The model under review builds one solid part; all positions refer to its coordinate system, in mm. A direction names the side the tool comes from. Coordinates: 2 decimals unless noted, no trailing zeros. Write each loop counter-clockwise with the first axis right and the second up, starting at its lowest first coordinate (ties: lowest second). Pieces come first, ordered by that corner, then holes. Notation, with made-up numbers: (33.25, 50.5) - (82.25, 50.5) arc R26 ccw to (82.25, 85.5) - close; hole circle Ø10 at (-35, 71.5). An arc over 180 degrees is marked (long way). Return JSON: item names as keys, results as strings. Group by question number.
(1) For pin 1 Ø1 at (x, z) = (5.5, 4) entering from -Y; pin 2 Ø1.5 at (x, z) = (-4, 5) entering from -Y; pin 3 Ø1.8 at (y, z) = (0, 1.5) entering from +X, all flat-tipped, find the tip position at first contact; note any pin that passes through.
(2) We need section D-D on x = 10.75. State the section outline as (y, z) points, then the cut area to 3 significant figures.
(3) Draft analysis for pull direction Y (two halves, no side actions). For faces 1 (the face through (6, -13, 0)), 2 (the face through (3.715, -19.396, 2.958)), 3 (the face through (15.62, -31.28, 3.04)), 4 (the face through (5.14, -47.3, 2.96)), state which applies: released by +Y, released by -Y, zero draft, split by the parting line, or undercut.
(4) We need section C-C on z = 1.05. State the section outline as (x, y) points.
(5) To check wall thickness, follow L1, parallel to Y at x = -1.25, z = 0.3; L2, parallel to X at y = -0.5, z = 0.7; L3, parallel to X at y = -13.5, z = 4. State the ranges of each line that lie inside material, in increasing order. Write a range as from..to.
(6) We need section A-A on x = 4.5. State the section outline as (y, z) points.
(7) Tool access review of faces 5 (the face through (3.93, -41.9, 2.96)), 6 (the face through (6, -13, 6)), 7 (the face through (0, 1.778, 3)): name each direction out of +Z, -Z, +X, -X, +Y, -Y from which nothing blocks a thin tool from reaching the whole face with its end or side.
(8) We need section B-B on y = 0. State the section outline as (x, z) points, then the cut area to 3 significant figures.
Autodesk Fusion 360 part; units mm, degrees
sketch "Sketch1" plane through (0, 0, 0) normal (0, 0, 1) x (1, 0, 0)
  circle A0 centre (0, 0) radius 10
  line L0 (-1.778, 1.778) -> (1.778, 1.778)
  line L1 (1.778, 1.778) -> (1.778, -1.778)
  line L2 (1.778, -1.778) -> (-1.778, -1.778)
  line L3 (-1.778, -1.778) -> (-1.778, 1.778)
  line L4 (-1.778, 1.778) -> (1.778, -1.778) construction
  line L5 (1.778, 1.778) -> (-1.778, -1.778) construction
  line L6 (0, 10) -> (0, -50.96)
  line L7 (0, -50.96) -> (11.2783, -42.9344)
  line L8 (0, -50.96) -> (8.4708, -31.4235)
  line L9 (9.8281, 1.8461) -> (16.0511, -31.2832)
  line L10 (11.2783, -42.9344) -> (16.0511, -31.2832)
  line L11 (8.4708, -31.4235) -> (0, -10)
  point P0 (-10, 0)
  point P1 (0, 10)
  dimension "d1" = 20
  dimension "d5" = 3.556
  dimension "d14" = 60.96
extrude "Extrude1" add sketch "Sketch1" along normal blind 6 contours A0 L0 L1 L2 L6 | A0 L7 L8 L9 L10 L11 | A0 L0 L2 L3 L6
fillet "Fillet4" radius 7.5 1 edges at (8.4708, -31.4235, 3)
fillet "Fillet5" radius 10 2 edges at (16.0511, -31.2832, 3) (11.2783, -42.9344, 3)
fillet "Fillet6" radius 0.5 1 edges at (0, -50.96, 3)
Ans:
{
 "1": {"pin 1": "y = -47.4", "pin 2": "y = -9.46", "pin 3": "x = 10.34"},
 "2": {"outline": "(-42.93, 0) - (-3.06, 0) - (-3.06, 6) - (-42.93, 6) - close", "area": "239 mm²"},
 "3": {"face 1": "zero draft", "face 2": "undercut", "face 3": "split by the parting line", "face 4": "released by -Y"},
 "4": {"outline": "(0, -10) - (7.33, -28.53) arc R7.5 cw to (7.23, -34.27) - (0.71, -49.31) arc R0.5 ccw to (1.46, -49.92) - (8.92, -44.61) arc R10 ccw to (12.38, -40.26) - (14.93, -34.02) arc R10 ccw to (15.51, -28.38) - (9.83, 1.85) arc R10 ccw (long way) to start; hole (-1.78, -1.78) - (1.78, -1.78) - (1.78, 1.78) - (-1.78, 1.78) - close"},
 "5": {"L1": "-9.92..-1.78, 1.78..9.92", "L2": "-9.99..-1.78, 1.78..10.27", "L3": "1.38..12.71"},
 "6": {"outline": "(-47.76, 0) - (-40.58, 0) - (-40.58, 6) - (-47.76, 6) - close; (-21.38, 0) - (8.93, 0) - (8.93, 6) - (-21.38, 6) - close"},
 "7": {"face 5": "+Z, -Z, -X", "face 6": "+Z, +X, -X, +Y, -Y", "face 7": "+Z, -Z"},
 "8": {"outline": "(-10, 0) - (-1.78, 0) - (-1.78, 6) - (-10, 6) - close; (1.78, 0) - (10.17, 0) - (10.17, 6) - (1.78, 6) - close", "area": "99.7 mm²"}
}
